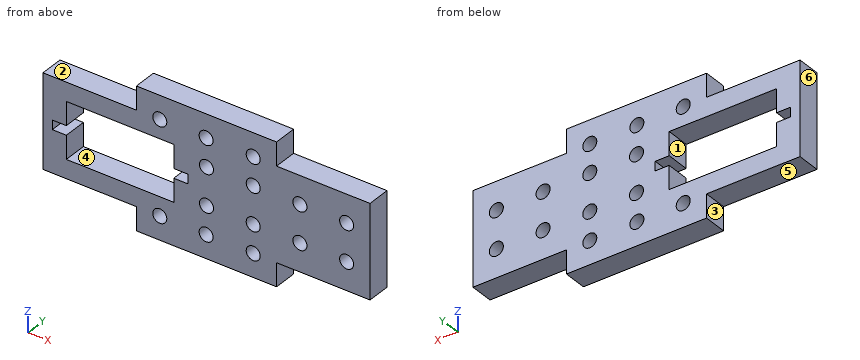
```python
from build123d import *

# Parameters (mm, degrees)
SKETCH_1_R      = 1.5
EXTRUDE_1_DEPTH = 5


with BuildPart() as part:
    # 草图1 → 凸台-拉伸1 (new body)
    with BuildSketch(Plane(origin=(0, 0, 0), x_dir=(1, 0, 0), z_dir=(0, 1, 0))):
        Polygon((50, 20), (70, 20), (70, 0), (50, 0), (50, -5), (20, -5), (20, 0), (0, 0), (0, 20), (20, 20), (20, 25), (50, 25), align=None)
        with Locations(Location((25, 20, 0), (0, 0, 270))):
            Circle(SKETCH_1_R, mode=Mode.SUBTRACT)
        with Locations(Location((34.920753824, 20, 0), (0, 0, 270))):
            Circle(SKETCH_1_R, mode=Mode.SUBTRACT)
        with Locations(Location((45, 20, 0), (0, 0, 270))):
            Circle(SKETCH_1_R, mode=Mode.SUBTRACT)
        with Locations(Location((35, 14, 0), (0, 0, 270))):
            Circle(SKETCH_1_R, mode=Mode.SUBTRACT)
        with Locations(Location((45, 14, 0), (0, 0, 270))):
            Circle(SKETCH_1_R, mode=Mode.SUBTRACT)
        with Locations(Location((35, 6, 0), (0, 0, 270))):
            Circle(SKETCH_1_R, mode=Mode.SUBTRACT)
        with Locations(Location((34.920753824, 0, 0), (0, 0, 270))):
            Circle(SKETCH_1_R, mode=Mode.SUBTRACT)
        with Locations(Location((45, 0, 0), (0, 0, 270))):
            Circle(SKETCH_1_R, mode=Mode.SUBTRACT)
        with Locations(Location((45, 6, 0), (0, 0, 270))):
            Circle(SKETCH_1_R, mode=Mode.SUBTRACT)
        with Locations(Location((55, 14, 0), (0, 0, 270))):
            Circle(SKETCH_1_R, mode=Mode.SUBTRACT)
        with Locations(Location((55, 6, 0), (0, 0, 270))):
            Circle(SKETCH_1_R, mode=Mode.SUBTRACT)
        with Locations(Location((65, 14, 0), (0, 0, 270))):
            Circle(SKETCH_1_R, mode=Mode.SUBTRACT)
        with Locations(Location((65, 6, 0), (0, 0, 270))):
            Circle(SKETCH_1_R, mode=Mode.SUBTRACT)
        with Locations(Location((25, 0, 0), (0, 0, 270))):
            Circle(SKETCH_1_R, mode=Mode.SUBTRACT)
        Polygon((5, 16), (28, 16), (28, 11), (31, 11), (31, 9), (28, 9), (28, 4), (5, 4), (5, 9), (2, 9), (2, 11), (5, 11), align=None, mode=Mode.SUBTRACT)
    extrude(amount=EXTRUDE_1_DEPTH)


solid = part.part
```
CAD build for the part. Positions are in the model's coordinates, mm. Face numbers are marked on the shaded views. A direction names the side the tool comes from. Give positions to 0.01 mm unless a question says otherwise; leave off trailing zeros. Write each loop counter-clockwise with the first axis right and the second up, starting at its lowest first coordinate (ties: lowest second). Pieces come first, ordered by that corner, then holes. Notation, with made-up numbers: M -14,-18.5 L 17,-18.5 A32 cw 17,13.5 Z; hole C 58.5,-26.5 d2. An arc over 180 degrees is marked long. Return JSON: item names as keys, results as strings. Group by question number.
(1) Drill centre lines: L1, parallel to X at y = 3.15, z = -6; L2, parallel to Z at x = 65, y = 2.6; L3, parallel to X at y = 2.1, z = -19.5. Where is each one in solid material? Low to high. Write a range as [from, to].
(2) Band-saw the part on B-B (x = 14.5). Give the cut face in (y, z).
(3) Mould opens along X. For the marked faces 4, 5 and 6 say: pulls with the +X half, pulls with the -X half, needs draft (parallel to the pull), parting line crosses it, or undercut.
(4) Band-saw the part on C-C (x = 65). Give the cut face in (y, z).
(5) Band-saw the part on D-D (x = 21.5). Give the cut face in (y, z).
(6) 3-axis set-ups, long thin cutter, end or side, ignore diameter. For the marked faces 1, 2 and 3: which of +Z, -Z, +X, -X, +Y, -Y reach the whole face in a straight line?
(7) Flat gauge pins, fed straight in: pin 1 Ø3.5 at (x, z) = (35, -6) entering from +Y; pin 2 Ø2.5 at (x, y) = (64, 3.5) entering from +Z; pin 3 Ø1.5 at (y, z) = (2.5, 2.5) entering from -X; pin 4 Ø2 at (y, z) = (3, 1.5) entering from +X. Where does each tip first touch, or does it go through?
(8) Band-saw the part on A-A (z = -6). Give the cut face in (x, y).
Entries:
{
 "1": {"L1": "x = [0, 5], [28, 33.5], [36.5, 43.5], [46.5, 53.5], [56.5, 63.5], [66.5, 70]", "L2": "z = [-20, -15.5], [-12.5, -7.5], [-4.5, 0]", "L3": "x = [0, 23.59], [26.41, 33.51], [36.33, 43.59], [46.41, 70]"},
 "2": {"outline": "M 0,-20 L 5,-20 L 5,-16 L 0,-16 Z; M 0,-4 L 5,-4 L 5,0 L 0,0 Z"},
 "3": {"face 4": "undercut", "face 5": "needs draft", "face 6": "pulls with the -X half"},
 "4": {"outline": "M 0,-20 L 5,-20 L 5,-15.5 L 0,-15.5 Z; M 0,-12.5 L 5,-12.5 L 5,-7.5 L 0,-7.5 Z; M 0,-4.5 L 5,-4.5 L 5,0 L 0,0 Z"},
 "5": {"outline": "M 0,-25 L 5,-25 L 5,-16 L 0,-16 Z; M 0,-4 L 5,-4 L 5,5 L 0,5 Z"},
 "6": {"face 1": "+Y, -Y", "face 2": "+Z, -X, +Y, -Y", "face 3": "-Z, -X, +Y, -Y"},
 "7": {"pin 1": "stops at y = 5", "pin 2": "stops at z = 0", "pin 3": "stops at x = 20", "pin 4": "stops at x = 50"},
 "8": {"outline": "M 0,0 L 5,0 L 5,5 L 0,5 Z; M 28,0 L 33.5,0 L 33.5,5 L 28,5 Z; M 36.5,0 L 43.5,0 L 43.5,5 L 36.5,5 Z; M 46.5,0 L 53.5,0 L 53.5,5 L 46.5,5 Z; M 56.5,0 L 63.5,0 L 63.5,5 L 56.5,5 Z; M 66.5,0 L 70,0 L 70,5 L 66.5,5 Z"}
}
